Could you check a few things on this model? Use its own coordinates, in mm. Face numbers are marked on the shaded views. A direction names the side the tool comes from. Coordinates: 2 decimals unless noted, no trailing zeros. Order: outer loops, then holes, each group sorted by start corner. A loop starts at its lowest first (then second) coordinate and runs counter-clockwise, first axis right, second up. Notation, with made-up numbers: (83, -37.75) - (116, -37.75) arc R20 cw to (116, -22.75) - close; hole circle Ø2 at (30, 85). An arc over 180 degrees is marked (long way). Answer as a JSON object with one key per item and string values. Group by question number.
(1) We'd pull the mould along Z, two halves only. Please class the marked faces 3, 4, 5 and 6: pulls with the +Z half, pulls with the -Z half, needs draft (parallel to the pull), parting line crosses it, or undercut.
(2) Imagine slicing it at A-A, the plane z = 10. Write out the boundary of the cut face in (x, y) (3 decimals), and give its area (3 significant figures).
(3) Will these pins go through, and if not, where does the flat tip stop? P1, Ø5, axis at x = -5, y = 1.5, coming from the +Z side; P2, Ø2, axis at y = 4, z = 10.5, coming from the +X side; P3, Ø3, axis at y = 0.5, z = 21.5, coming from the -X side.
(4) Please list where these lines run through material, in increasing order: probe 1 along Z at (x, y) = (0, 2.65); probe 2 along Z at (x, y) = (0, 3.15); probe 3 along Z at (x, y) = (-6, 1).
(5) Which directions (+Z, -Z, +X, -X, +Y, -Y) give clear straight access to the entire face, cutting with the end or side of a thin tool? Please do the marked faces 1 and 2.
from build123d import *

# Parameters (mm, degrees)
SKETCH001_AS_DRAWN_R                 = 5
EXTRUDE001_DEPTH                     = 5
EXTRUDE001_ONTO_SKETCH001_ROLL_ANGLE = 90
FILLET_R                             = 7
POCKET_DEPTH                         = 2
REVOLVE_ANGLE                        = 180
REVOLVE_ONTO_SKETCH003_ROLL_ANGLE    = 90
POCKET001_DEPTH                      = 4
SKETCH005_R                          = 1.55
POCKET002_DEPTH                      = 2.693383
POCKET003_DEPTH                      = 9.758576


with BuildPart() as pocket:
    # Sketch001 as drawn → Extrude001 (new)
    with BuildSketch(Plane.XY):
        with BuildLine():
            Line((-7, 0), (7, 0))
            Line((7, 0), (7, 5))
            ThreePointArc((7, 5), (0, 35.598621), (-7, 5))
            Line((-7, 0), (-7, 5))
        make_face()
        with Locations((0, 19.498621)):
            Circle(SKETCH001_AS_DRAWN_R, mode=Mode.SUBTRACT)
        with BuildLine():
            ThreePointArc((-6.05, 29.977528), (-12.1, 19.498621), (-6.05, 9.019713))
            ThreePointArc((-6.05, 9.019713), (-3.932661, 9.587053), (-4.5, 11.704392))
            ThreePointArc((-4.5, 27.292849), (-9, 19.498621), (-4.5, 11.704392))
            ThreePointArc((-4.5, 27.292849), (-3.932661, 29.410189), (-6.05, 29.977528))
        make_face(mode=Mode.SUBTRACT)
        with BuildLine():
            ThreePointArc((4.5, 11.704392), (9, 19.498621), (4.5, 27.292849))
            ThreePointArc((6.05, 29.977528), (3.932661, 29.410189), (4.5, 27.292849))
            ThreePointArc((6.05, 9.019713), (12.1, 19.498621), (6.05, 29.977528))
            ThreePointArc((4.5, 11.704392), (3.932661, 9.587053), (6.05, 9.019713))
        make_face(mode=Mode.SUBTRACT)
    extrude(amount=-EXTRUDE001_DEPTH)


with BuildPart() as pocket_1:
    # Extrude001 onto Sketch001 roll: moved
    add(pocket.part.rotate(Axis((0, 0, 0), (1, 0, 0)), EXTRUDE001_ONTO_SKETCH001_ROLL_ANGLE))


with BuildPart() as pocket_2:
    # Extrude001 onto Sketch001 placement: moved
    add(pocket_1.part)

    # Fillet
    fillet_edges = [pocket_2.edges().sort_by_distance(p)[0] for p in [
        (7, 2.5, 5),
        (-7, 2.5, 5),
    ]]
    fillet(fillet_edges, radius=FILLET_R)

    # Sketch002 → Pocket (cut)
    with BuildSketch(Plane(origin=(0, 5, 0), x_dir=(-1, 0, 0), z_dir=(0, 1, 0))):
        with BuildLine():
            ThreePointArc((-3.85, 26.167016), (-7.7, 19.498621), (-3.85, 12.830225))
            Line((-3.85, 12.830225), (-2.425, 12.007501))
            Line((-2.425, 12.007501), (-2.425, 10.362053))
            Line((-2.425, 10.362053), (-2.425, 8.716604))
            Line((-2.425, 8.716604), (-3.85, 7.89388))
            Line((-3.85, 7.89388), (-5.275, 7.071156))
            Line((-5.275, 7.071156), (-6.7, 7.89388))
            ThreePointArc((-6.7, 31.103361), (-13.4, 19.498621), (-6.7, 7.89388))
            Line((-6.7, 31.103361), (-5.275, 31.926085))
            Line((-5.275, 31.926085), (-3.85, 31.103361))
            Line((-3.85, 31.103361), (-2.425, 30.280637))
            Line((-2.425, 30.280637), (-2.425, 28.635189))
            Line((-2.425, 28.635189), (-2.425, 26.98974))
            Line((-2.425, 26.98974), (-3.85, 26.167016))
        make_face()
        with BuildLine():
            ThreePointArc((3.85, 12.830225), (7.7, 19.498621), (3.85, 26.167016))
            Line((3.85, 26.167016), (2.424998, 26.989738))
            Line((2.424998, 26.989738), (2.425, 28.635187))
            Line((2.425, 28.635187), (2.425002, 30.280636))
            Line((2.425002, 30.280636), (3.850002, 31.103362))
            Line((3.850002, 31.103362), (5.275001, 31.926088))
            Line((5.275001, 31.926088), (6.7, 31.103361))
            ThreePointArc((6.7, 7.89388), (13.4, 19.498621), (6.7, 31.103361))
            Line((5.275, 7.071157), (6.7, 7.89388))
            Line((3.85, 7.89388), (5.275, 7.071157))
            Line((2.425, 8.716604), (3.85, 7.89388))
            Line((2.425, 10.362052), (2.425, 8.716604))
            Line((2.425, 12.0075), (2.425, 10.362052))
            Line((3.85, 12.830225), (2.425, 12.0075))
        make_face()
    extrude(amount=-POCKET_DEPTH, mode=Mode.SUBTRACT)


with BuildPart() as pocket003:
    # Sketch003 as drawn → Revolve (revolve)
    with BuildSketch(Plane.XY):
        with BuildLine():
            ThreePointArc((-7, 1.124454), (-7.727163, 4.231143), (-9.757576, 6.692383))
            Line((0, 6.692383), (-9.757576, 6.692383))
            Line((0, 0), (0, 6.692383))
            Line((-7, 0), (0, 0))
            Line((-7, 1.124454), (-7, 0))
        make_face()
    revolve(axis=Axis((0, 0, 0), (0, 1, 0)), revolution_arc=REVOLVE_ANGLE)


with BuildPart() as pocket003_1:
    # Revolve onto Sketch003 roll: moved
    add(pocket003.part.rotate(Axis((0, 0, 0), (1, 0, 0)), REVOLVE_ONTO_SKETCH003_ROLL_ANGLE))


with BuildPart() as pocket003_2:
    # Revolve onto Sketch003 placement: moved
    add(pocket003_1.part)

    # Fusion: union Pocket
    add(pocket_2.part)

    # Sketch004 → Pocket001 (cut)
    with BuildSketch(Plane.XY.offset(6.692383)):
        Polygon((2.641377, -1.525), (2.641377, 1.525), (0, 3.05), (-2.641377, 1.525), (-2.641377, -1.525), (0, -3.05), align=None)
    extrude(amount=-POCKET001_DEPTH, mode=Mode.SUBTRACT)

    # Sketch005 → Pocket002 (cut, through all)
    with BuildSketch(Plane.XY.offset(2.692383)):
        Circle(SKETCH005_R)
    extrude(amount=-POCKET002_DEPTH, mode=Mode.SUBTRACT)

    # Sketch006 → Pocket003 (cut, through all)
    with BuildSketch(Plane.XZ):
        with BuildLine():
            Line((-9.757576, 6.692383), (9.757576, 6.692383))
            ThreePointArc((-9.757576, 6.692383), (0, 3.398621), (9.757576, 6.692383))
        make_face()
    extrude(amount=POCKET003_DEPTH, mode=Mode.SUBTRACT)


solid = pocket003_2.part
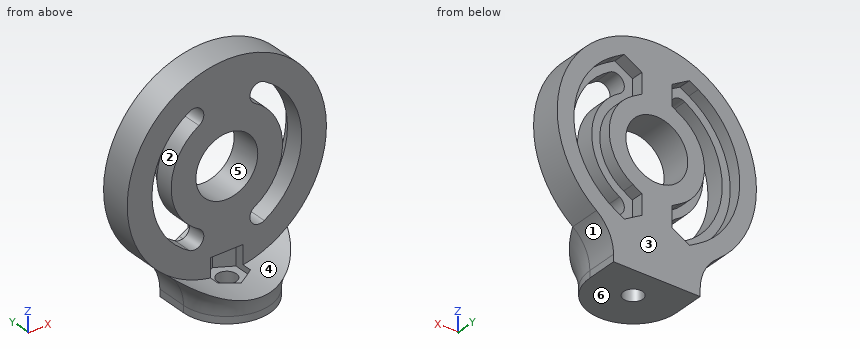
Result set:
{
 "1": {"face 3": "needs draft", "face 4": "pulls with the +Z half", "face 5": "undercut", "face 6": "pulls with the -Z half"},
 "2": {"outline": "(-12.999, 0) - (-7.496, 0) - (-7.496, 3) - (-9.452, 3) - (-9.452, 5) - (-12.999, 5) - close; (-3.768, 0) - (3.768, 0) - (3.768, 3) - (2.425, 3) - (2.425, 5) - (-2.425, 5) - (-2.425, 3) - (-3.768, 3) - close; (7.496, 0) - (12.999, 0) - (12.999, 5) - (9.452, 5) - (9.452, 3) - (7.496, 3) - close", "area": "79.5 mm^2"},
 "3": {"P1": "stops at z = 35.4", "P2": "stops at x = 13.97", "P3": "stops at x = -16.09"},
 "4": {"probe 1": "z = 0 to 2.69, 6.69 to 14.5, 24.5 to 35.6", "probe 2": "z = 0 to 14.5, 24.5 to 35.6", "probe 3": "z = 0 to 8.99, 12.79 to 26.21, 30.01 to 34.44"},
 "5": {"face 1": "-Z, +X, +Y, -Y", "face 2": "+Y, -Y"}
}
